from build123d import *

# Parameters (mm, degrees)
F1_DEPTH = 20
F0_W     = 8
F0_H     = 8
F2_DEPTH = 4
F3_DEPTH = 8


with BuildPart() as f1:
    # F0 (on Top) → F1 (new body)
    with BuildSketch(Plane.XY):
        with BuildLine():
            Line((23.9531163031, -38.0952519268), (27.5699483395, -41.7120839632))
            ThreePointArc((27.5699483395, -41.7120839632), (31.6227766017, -38.7298334621), (35.3553390593, -35.3553390593))
            Line((35.3553390593, -35.3553390593), (31.8198051534, -31.8198051534))
            ThreePointArc((31.8198051534, -31.8198051534), (28.0624304008, -35.1781181987), (23.9531163031, -38.0952519268))
        make_face()
        with BuildLine():
            ThreePointArc((35.3553390593, -35.3553390593), (38.7298334621, -31.6227766017), (41.7120839632, -27.5699483395))
            Line((41.7120839632, -27.5699483395), (38.0952519268, -23.9531163031))
            ThreePointArc((38.0952519268, -23.9531163031), (35.1781181987, -28.0624304008), (31.8198051534, -31.8198051534))
            Line((31.8198051534, -31.8198051534), (35.3553390593, -35.3553390593))
        make_face()
        with BuildLine():
            ThreePointArc((41.7120839632, -27.5699483395), (47.883213124, -14.3943704593), (50, 0))
            ThreePointArc((50, 0), (-44.0369016677, 23.6801877423), (27.5699483395, -41.7120839632))
            Line((27.5699483395, -41.7120839632), (23.9531163031, -38.0952519268))
            ThreePointArc((23.9531163031, -38.0952519268), (14.3755356179, -42.6420446941), (4, -44.821869662))
            ThreePointArc((4, -44.821869662), (0, -45), (-4, -44.821869662))
            ThreePointArc((-4, -44.821869662), (-31.8198051534, -31.8198051534), (-44.821869662, -4))
            ThreePointArc((-44.821869662, -4), (-45, 0), (-44.821869662, 4))
            ThreePointArc((-44.821869662, 4), (-31.8198051534, 31.8198051534), (-4, 44.821869662))
            ThreePointArc((-4, 44.821869662), (0, 45), (4, 44.821869662))
            ThreePointArc((4, 44.821869662), (31.8198051534, 31.8198051534), (44.821869662, 4))
            ThreePointArc((44.821869662, 4), (44.9554453587, 2.0019821688), (45, 0))
            ThreePointArc((45, 0), (44.9554453587, -2.0019821688), (44.821869662, -4))
            ThreePointArc((44.821869662, -4), (42.6420446941, -14.3755356179), (38.0952519268, -23.9531163031))
            Line((38.0952519268, -23.9531163031), (41.7120839632, -27.5699483395))
        make_face()
    extrude(amount=F1_DEPTH)

    # F0 (on Top) → F2 (join)
    with BuildSketch(Plane.XY):
        with BuildLine():
            Line((4, 14.4568322948), (4, 44.821869662))
            ThreePointArc((4, 44.821869662), (0, 45), (-4, 44.821869662))
            Line((-4, 44.821869662), (-4, 14.4568322948))
            ThreePointArc((-4, 14.4568322948), (0, 15), (4, 14.4568322948))
        make_face()
        with BuildLine():
            Line((-4, 4), (4, 4))
            Line((4, 4), (4, 6.25))
            Line((4, 6.25), (4, 14.4568322948))
            ThreePointArc((4, 14.4568322948), (0, 15), (-4, 14.4568322948))
            Line((-4, 14.4568322948), (-4, 6.25))
            Line((-4, 6.25), (-4, 4))
        make_face()
        with BuildLine():
            Line((14.4568322948, -4), (44.821869662, -4))
            ThreePointArc((44.821869662, -4), (44.9554453587, -2.0019821688), (45, 0))
            ThreePointArc((45, 0), (44.9554453587, 2.0019821688), (44.821869662, 4))
            Line((44.821869662, 4), (14.4568322948, 4))
            ThreePointArc((14.4568322948, 4), (14.8635877974, 2.0183552187), (15, 0))
            ThreePointArc((15, 0), (14.8635877974, -2.0183552187), (14.4568322948, -4))
        make_face()
        with BuildLine():
            Line((6.2500000127, 4), (14.4568322948, 4))
            ThreePointArc((14.4568322948, 4), (10.6066017178, 10.6066017178), (4, 14.4568322948))
            Line((4, 14.4568322948), (4, 6.25))
            ThreePointArc((4, 6.25), (6.25, 8.5), (8.5, 6.25))
            ThreePointArc((8.5, 6.25), (7.8409902621, 4.6590097468), (6.2500000127, 4))
        make_face()
        with BuildLine():
            Line((6.2499999791, -4), (14.4568322948, -4))
            ThreePointArc((14.4568322948, -4), (14.8635877974, -2.0183552187), (15, 0))
            ThreePointArc((15, 0), (14.8635877974, 2.0183552187), (14.4568322948, 4))
            Line((14.4568322948, 4), (6.2500000127, 4))
            Line((6.2500000127, 4), (4, 4))
            Line((4, 4), (4, -4))
            Line((4, -4), (6.2499999791, -4))
        make_face()
        with BuildLine():
            Line((4, 6.25), (4, 4))
            Line((4, 4), (6.2500000127, 4))
            ThreePointArc((6.2500000127, 4), (4.6590097468, 4.6590097379), (4, 6.25))
        make_face()
        Rectangle(F0_W, F0_H)
        with BuildLine():
            ThreePointArc((-14.4568322948, 4), (-15, 0), (-14.4568322948, -4))
            Line((-14.4568322948, -4), (-6.2500000209, -4))
            Line((-6.2500000209, -4), (-4, -4))
            Line((-4, -4), (-4, 4))
            Line((-4, 4), (-6.2499999873, 4))
            Line((-6.2499999873, 4), (-14.4568322948, 4))
        make_face()
        with BuildLine():
            ThreePointArc((-4, 14.4568322948), (-10.6066017178, 10.6066017178), (-14.4568322948, 4))
            Line((-14.4568322948, 4), (-6.2499999873, 4))
            ThreePointArc((-6.2499999873, 4), (-7.8409902621, 7.8409902532), (-4, 6.25))
            Line((-4, 6.25), (-4, 14.4568322948))
        make_face()
        with BuildLine():
            ThreePointArc((-14.4568322948, -4), (-10.6066017178, -10.6066017178), (-4, -14.4568322948))
            Line((-4, -14.4568322948), (-4, -6.25))
            ThreePointArc((-4, -6.25), (-7.8409902503, -7.8409902651), (-6.2500000209, -4))
            Line((-6.2500000209, -4), (-14.4568322948, -4))
        make_face()
        with BuildLine():
            Line((4, -4), (4, -6.25))
            ThreePointArc((4, -6.25), (4.1712710518, -5.3889622772), (4.6590097423, -4.6590097423))
            Line((4.6590097423, -4.6590097423), (4, -4))
        make_face()
        with BuildLine():
            ThreePointArc((4, -14.4568322948), (7.5527658715, -12.9597734429), (10.6066017178, -10.6066017178))
            Line((10.6066017178, -10.6066017178), (7.8409902577, -7.8409902577))
            ThreePointArc((7.8409902577, -7.8409902577), (5.3889622772, -8.3287289482), (4, -6.25))
            Line((4, -6.25), (4, -14.4568322948))
        make_face()
        with BuildLine():
            ThreePointArc((-4, -44.821869662), (0, -45), (4, -44.821869662))
            Line((4, -44.821869662), (4, -14.4568322948))
            ThreePointArc((4, -14.4568322948), (0, -15), (-4, -14.4568322948))
            Line((-4, -14.4568322948), (-4, -44.821869662))
        make_face()
        with BuildLine():
            ThreePointArc((-44.821869662, 4), (-45, 0), (-44.821869662, -4))
            Line((-44.821869662, -4), (-14.4568322948, -4))
            ThreePointArc((-14.4568322948, -4), (-15, 0), (-14.4568322948, 4))
            Line((-14.4568322948, 4), (-44.821869662, 4))
        make_face()
        with BuildLine():
            ThreePointArc((-4, -14.4568322948), (0, -15), (4, -14.4568322948))
            Line((4, -14.4568322948), (4, -6.25))
            Line((4, -6.25), (4, -4))
            Line((4, -4), (-4, -4))
            Line((-4, -4), (-4, -6.25))
            Line((-4, -6.25), (-4, -14.4568322948))
        make_face()
        with BuildLine():
            ThreePointArc((-6.2500000209, -4), (-4.6590097497, -4.6590097349), (-4, -6.25))
            Line((-4, -6.25), (-4, -4))
            Line((-4, -4), (-6.2500000209, -4))
        make_face()
        with BuildLine():
            ThreePointArc((-4, 6.25), (-4.6590097379, 4.6590097468), (-6.2499999873, 4))
            Line((-6.2499999873, 4), (-4, 4))
            Line((-4, 4), (-4, 6.25))
        make_face()
        with BuildLine():
            Line((7.8409902577, -7.8409902577), (10.6066017178, -10.6066017178))
            ThreePointArc((10.6066017178, -10.6066017178), (12.9597734429, -7.5527658715), (14.4568322948, -4))
            Line((14.4568322948, -4), (6.2499999791, -4))
            ThreePointArc((6.2499999791, -4), (7.8409902503, -4.6590097349), (8.5, -6.25))
            ThreePointArc((8.5, -6.25), (8.3287289482, -7.1110377228), (7.8409902577, -7.8409902577))
        make_face()
        with BuildLine():
            ThreePointArc((4.6590097423, -4.6590097423), (5.3889622675, -4.1712710559), (6.2499999791, -4))
            Line((6.2499999791, -4), (4, -4))
            Line((4, -4), (4.6590097423, -4.6590097423))
        make_face()
    extrude(amount=F2_DEPTH)

    # F0 (on Top) → F3 (cut)
    with BuildSketch(Plane.XY):
        with BuildLine():
            ThreePointArc((35.3553390593, -35.3553390593), (38.7298334621, -31.6227766017), (41.7120839632, -27.5699483395))
            Line((41.7120839632, -27.5699483395), (38.0952519268, -23.9531163031))
            ThreePointArc((38.0952519268, -23.9531163031), (35.1781181987, -28.0624304008), (31.8198051534, -31.8198051534))
            Line((31.8198051534, -31.8198051534), (35.3553390593, -35.3553390593))
        make_face()
        with BuildLine():
            Line((23.9531163031, -38.0952519268), (27.5699483395, -41.7120839632))
            ThreePointArc((27.5699483395, -41.7120839632), (31.6227766017, -38.7298334621), (35.3553390593, -35.3553390593))
            Line((35.3553390593, -35.3553390593), (31.8198051534, -31.8198051534))
            ThreePointArc((31.8198051534, -31.8198051534), (28.0624304008, -35.1781181987), (23.9531163031, -38.0952519268))
        make_face()
    extrude(amount=F3_DEPTH, mode=Mode.SUBTRACT)


solid = f1.part
Model file for the job. Use its own axes, mm. A direction names the side the tool comes from. Coordinates: 2 decimals unless noted, no trailing zeros. Order: outer loops, then holes, each group sorted by start corner. A loop starts at its lowest first (then second) coordinate and runs counter-clockwise, first axis right, second up. Notation, with made-up numbers: (49, 86) -> (73, 86) arc R24 cw to (73, 121) -> close; hole circle Ø5 at (84, -11). An arc over 180 degrees is marked (long way). Return JSON: item names as keys, results as strings. Group by question number.
Item 1: Wall check: line 1 along X through (y, z) = (-6.25, 2.8); line 2 along X through (y, z) = (19, 18); line 3 along X through (y, z) = (25, 19). Give the ranges that are in metal, low to high. Write a range as [from, to].
Item 2: Saw through at B-B on x = -12. Write the cut outline in (y, z), then the cut area to 3 significant figures.
Item 3: Saw through at D-D on x = 0. Write the cut outline in (y, z), then the cut area to 3 significant figures.
Item 4: Saw through at C-C on y = 36.5. Write the cut outline in (x, z).
Item 5: Saw through at A-A on z = 18.25. Write the cut outline in (x, y), then the cut area to 3 significant figures.
Item 6: Flat gauge pins, fed straight in: P1, Ø8, axis at x = -7, z = 16.5, coming from the -Y side; P2, Ø2, axis at x = -37, z = 3.5, coming from the -Y side; P3, Ø1.2, axis at y = 31.5, z = 2, coming from the -X side; P4, Ø6, axis at x = -6.25, y = -6.25, coming from the -Z side. Where does each tip first touch, or does it go through?
Item 7: Tool access for faces 1 (the flat face through (33, -33, 8)), 2 (the flat face through (39.93, -25.79, 3.94)), 3 (the flat face through (0, 0, 4)), 4 (the flat face through (30, 4, 2)): list every direction of +Z, -Z, +X, -X, +Y, -Y with a clear straight run to the whole face (end or side of a thin tool).
Item 8: Pull direction X, two halves, no side cores. Call faces 5 (the flat face through (-1, 1, 0)), 6 (the flat face through (-4, -29, 2)), 7 (the flat face through (25.74, -39.88, 3.94)): pulls with the +X half, pulls with the -X half, needs draft (parallel to the pull), parting line crosses it, or undercut.
Values found:
{
 "1": {"line 1": "x = [-49.61, -44.56], [-13.64, -8.5], [-4, 4], [8.5, 13.64], [44.56, 49.61]", "line 2": "x = [-46.25, -40.79], [40.79, 46.25]", "line 3": "x = [-43.3, -37.42], [37.42, 43.3]"},
 "2": {"outline": "(-48.54, 0) -> (-43.37, 0) -> (-43.37, 20) -> (-48.54, 20) -> close; (-9, 0) -> (9, 0) -> (9, 4) -> (-9, 4) -> close; (43.37, 0) -> (48.54, 0) -> (48.54, 20) -> (43.37, 20) -> close", "area": "279 mm2"},
 "3": {"outline": "(-50, 0) -> (50, 0) -> (50, 20) -> (45, 20) -> (45, 4) -> (-45, 4) -> (-45, 20) -> (-50, 20) -> close", "area": "560 mm2"},
 "4": {"outline": "(-34.17, 0) -> (-26.32, 0) -> (-26.32, 20) -> (-34.17, 20) -> close; (-4, 0) -> (4, 0) -> (4, 4) -> (-4, 4) -> close; (26.32, 0) -> (34.17, 0) -> (34.17, 20) -> (26.32, 20) -> close"},
 "5": {"outline": "circle Ø100 at (0, 0); hole circle Ø90 at (0, 0)", "area": "1,490 mm2"},
 "6": {"P1": "stops at y = -49.91", "P2": "stops at y = -34.7", "P3": "stops at x = -39.31", "P4": "stops at z = 0"},
 "7": {"face 1": "-Z", "face 2": "-Z, -Y", "face 3": "+Z", "face 4": "+Z, -Z"},
 "8": {"face 5": "needs draft", "face 6": "undercut", "face 7": "pulls with the +X half"}
}
